Model file for the job. Use its own axes, mm. Round coordinates to 2 decimals unless told otherwise and drop trailing zeros. Order: outer loops, then holes, each group sorted by start corner. A loop starts at its lowest first (then second) coordinate and runs counter-clockwise, first axis right, second up. Notation, with made-up numbers: (-24.5, 39) -> (16.5, 39) arc R27 cw to (16.5, 78) -> close; hole circle Ø6 at (-5.75, 42.5). An arc over 180 degrees is marked (long way). Put each result on its own line as item: value. Start each with the question number.
Q1. Cut at B-B, the plane y = 1.75. List the corners of the cut face in (x, z).
Q2. Probe L1, parallel to Z at x = 0, y = 1; L2, parallel to X at y = 3.3, z = -80; L3, parallel to Z at x = -0.5, y = 2.2. List the from-to ranges inside material, lowest first.
Q3. Pull direction X, two halves, no side cores. Call faces 1 (the face through (0, 5, -41)), 2 (the face through (-1.15, 2.46, -77.78)), 3 (the face through (0, 2, 5)): released by +X, released by -X, zero draft, split by the parting line, or undercut.
Q4. Cut at A-A, the plane x = 0. List the corners of the cut face in (y, z).
from build123d import *

# Parameters (mm, degrees)
BOSS_EXTRUDE3_DEPTH = 5


with BuildPart() as part:
    # Sketch1 → Boss-Extrude3 (new body)
    with BuildSketch(Plane(origin=(0, 0, 0), x_dir=(1, 0, 0), z_dir=(0, 1, 0))):
        with BuildLine():
            ThreePointArc((-5, 0), (0, -5), (5, 0))
            Line((5, 0), (2.404574114, 0))
            ThreePointArc((2.404574114, 0), (0, -2.404574114), (-2.404574114, 0))
            Line((-2.404574114, 0), (-5, 0))
        make_face()
        with BuildLine():
            Line((2.404574114, 0), (5, 0))
            ThreePointArc((5, 0), (0, 5), (-5, 0))
            Line((-5, 0), (-2.404574114, 0))
            ThreePointArc((-2.404574114, 0), (0, 2.404574114), (2.404574114, 0))
        make_face()
        with BuildLine():
            ThreePointArc((-5, 0), (0, 5), (5, 0))
            Line((5, 0), (5, 80))
            ThreePointArc((5, 80), (0, 75), (-5, 80))
            Line((-5, 80), (-5, 0))
        make_face()
        with BuildLine():
            ThreePointArc((-5, 80), (0, 75), (5, 80))
            Line((5, 80), (2.5, 80))
            ThreePointArc((2.5, 80), (0, 77.5), (-2.5, 80))
            Line((-2.5, 80), (-5, 80))
        make_face()
        with BuildLine():
            Line((2.5, 80), (5, 80))
            ThreePointArc((5, 80), (0, 85), (-5, 80))
            Line((-5, 80), (-2.5, 80))
            ThreePointArc((-2.5, 80), (0, 82.5), (2.5, 80))
        make_face()
    extrude(amount=BOSS_EXTRUDE3_DEPTH)


solid = part.part
Ans:
1. outline: (-5, -80) arc R5 ccw to (5, -80) -> (5, 0) arc R5 ccw to (-5, 0) -> close; hole circle Ø5 at (0, -80); hole circle Ø4.81 at (0, 0)
2. L1: z = -85 to -82.5, -77.5 to -2.4, 2.4 to 5
2. L2: x = -5 to -2.5, 2.5 to 5
2. L3: z = -84.97 to -82.45, -77.55 to -2.35, 2.35 to 4.97
3. face 1: zero draft
3. face 2: undercut
3. face 3: split by the parting line
4. outline: (0, -85) -> (5, -85) -> (5, -82.5) -> (0, -82.5) -> close; (0, -77.5) -> (5, -77.5) -> (5, -2.4) -> (0, -2.4) -> close; (0, 2.4) -> (5, 2.4) -> (5, 5) -> (0, 5) -> close
